Geometry check sheet. Reference: the model listing, model coordinates, mm. Face numbers are marked on the shaded views. A direction names the side the tool comes from. Give positions to 0.01 mm unless a question says otherwise; leave off trailing zeros. Write each loop counter-clockwise with the first axis right and the second up, starting at its lowest first coordinate (ties: lowest second). Pieces come first, ordered by that corner, then holes. Notation, with made-up numbers: (33, 75) - (83, 75) arc R36 ccw to (83, 109) - close; hole circle Ø7 at (60, 34.25). An arc over 180 degrees is marked (long way). Use a Markdown table: item, result.
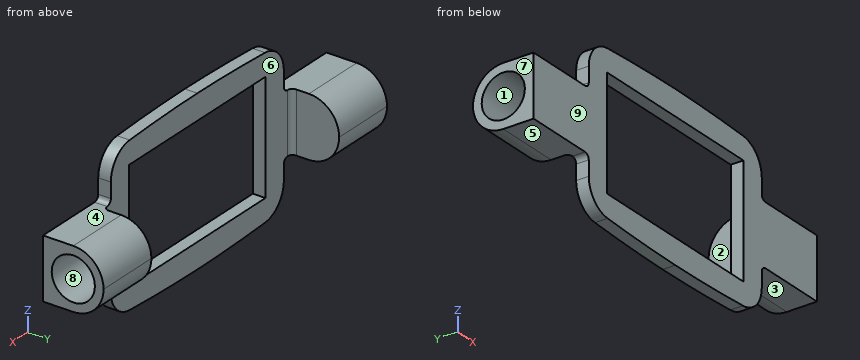
```python
from build123d import *

# Parameters (mm, degrees)
SKETCH2_W           = 93.98
SKETCH2_H           = 55.88
BOSS_EXTRUDE1_DEPTH = 6.35
SKETCH3_W           = 33.02
SKETCH3_H           = 30.48
BOSS_EXTRUDE2_DEPTH = 24.13
FILLET1_R           = 2.54
SKETCH4_R           = 10.8585
CUT_EXTRUDE1_DEPTH  = 25.4
CUT_EXTRUDE2_START  = -25.4
SKETCH5_R           = 10.8585
CUT_EXTRUDE2_DEPTH  = 25.4
FILLET2_R           = 2.54
FILLET3_R           = 15.24


with BuildPart() as part:
    # Sketch2 → Boss-Extrude1 (new body)
    with BuildSketch(Plane(origin=(0, 0, 0), x_dir=(1, 0, 0), z_dir=(0, 1, 0))):
        with BuildLine():
            ThreePointArc((-93.688069253, -11.244332686), (-70.349230661, -12.298232488), (-46.99, -12.696270789))
            ThreePointArc((-46.99, -12.696270789), (-23.630769339, -12.298232488), (-0.291930747, -11.244332686))
            ThreePointArc((-0.291930747, -11.244332686), (8.940138318, -6.930983214), (12.7, 2.54))
            Line((12.7, 2.54), (12.7, 12.7))
            Line((12.7, 12.7), (50.8, 12.7))
            Line((50.8, 12.7), (50.8, 43.18))
            Line((50.8, 43.18), (12.7, 43.18))
            Line((12.7, 43.18), (12.7, 53.34))
            ThreePointArc((12.7, 53.34), (8.940138318, 62.810983214), (-0.291930747, 67.124332686))
            ThreePointArc((-0.291930747, 67.124332686), (-23.630769339, 68.178232488), (-46.99, 68.576270789))
            ThreePointArc((-46.99, 68.576270789), (-70.349230661, 68.178232488), (-93.688069253, 67.124332686))
            ThreePointArc((-93.688069253, 67.124332686), (-102.920138318, 62.810983214), (-106.68, 53.34))
            Line((-106.68, 53.34), (-106.68, 43.18))
            Line((-106.68, 43.18), (-144.78, 43.18))
            Line((-144.78, 43.18), (-144.78, 12.7))
            Line((-144.78, 12.7), (-106.68, 12.7))
            Line((-106.68, 12.7), (-106.68, 2.54))
            ThreePointArc((-106.68, 2.54), (-102.920138318, -6.930983214), (-93.688069253, -11.244332686))
        make_face()
        with Locations((-46.99, 27.94)):
            Rectangle(SKETCH2_W, SKETCH2_H, mode=Mode.SUBTRACT)
    extrude(amount=BOSS_EXTRUDE1_DEPTH)

    # Sketch3 → Boss-Extrude2 (add)
    with BuildSketch(Plane(origin=(0, 6.35, 0), x_dir=(1, 0, 0), z_dir=(0, 1, 0))):
        with Locations((34.29, 27.94)):
            Rectangle(SKETCH3_W, SKETCH3_H)
        with Locations((-128.27, 27.94)):
            Rectangle(SKETCH3_W, SKETCH3_H)
    extrude(amount=BOSS_EXTRUDE2_DEPTH)

    # Fillet1
    fillet1_edges = [part.edges().sort_by_distance(p)[0] for p in [
        (17.78, 6.35, -27.94),
        (-111.76, 6.35, -27.94),
    ]]
    fillet(fillet1_edges, radius=FILLET1_R)

    # Sketch4 → Cut-Extrude1 (cut)
    with BuildSketch(Plane(origin=(50.8, 0, 0), x_dir=(0, 0, -1), z_dir=(1, 0, 0))):
        with Locations((27.94, 15.24)):
            Circle(SKETCH4_R)
    extrude(amount=-CUT_EXTRUDE1_DEPTH, mode=Mode.SUBTRACT)

    # Sketch5 → Cut-Extrude2 (cut)
    with BuildSketch(Plane.ZY.offset(144.78).offset(CUT_EXTRUDE2_START)):
        with Locations(Location((-27.94, 15.24, 0), (0, 0, 180))):
            Circle(SKETCH5_R)
    extrude(amount=CUT_EXTRUDE2_DEPTH, mode=Mode.SUBTRACT)

    # Fillet2
    fillet2_edges = [part.edges().sort_by_distance(p)[0] for p in [
        (12.7, 3.175, -43.18),
        (12.7, 3.175, -12.7),
        (-106.68, 3.175, -43.18),
        (-106.68, 3.175, -12.7),
    ]]
    fillet(fillet2_edges, radius=FILLET2_R)

    # Fillet3
    fillet3_edges = [part.edges().sort_by_distance(p)[0] for p in [
        (34.29, 30.48, -43.18),
        (34.29, 30.48, -12.7),
        (-128.27, 30.48, -43.18),
        (-128.27, 30.48, -12.7),
    ]]
    fillet(fillet3_edges, radius=FILLET3_R - 0.0001)  # a hair under: the kernel refuses the full size


solid = part.part
```
1) Material ranges on L1, parallel to X at y = 9.5, z = -25; L2, parallel to Y at x = 34.25, z = -27.94; L3, parallel to Z at x = 39, y = 15, recorded low to high. Write a range as from..to.
Working result:
| item | result |
|---|---|
| L1 | x = -119.38..-111.76, 17.78..25.4 |
| L2 | y = 0..4.38, 26.1..30.48 |
| L3 | z = -43.18..-38.8, -17.08..-12.7 |
2) Section check D-D on x = -61. Record the boundary of the cut face in (y, z).
Working result:
| item | result |
|---|---|
| outline | (0, -68.42) - (6.35, -68.42) - (6.35, -55.88) - (0, -55.88) - close; (0, 0) - (6.35, 0) - (6.35, 12.54) - (0, 12.54) - close |
3) Mould release check, pull along Y, two halves, no side actions. Record for the marked faces 6, 7, 8 and 9: pulls with the +Y half, pulls with the -Y half, needs draft (parallel to the pull), parting line crosses it, or undercut.
Working result:
| item | result |
|---|---|
| face 6 | pulls with the +Y half |
| face 7 | needs draft |
| face 8 | undercut |
| face 9 | pulls with the -Y half |
4) Set-up check for the marked faces 1, 2, 3, 4 and 5: record each of +Z, -Z, +X, -X, +Y, -Y from which the full face is reachable in a straight line by a thin tool's end or side.
Working result:
| item | result |
|---|---|
| face 1 | -X |
| face 2 | +Z, -Z, +Y |
| face 3 | -Z, +X, +Y, -Y |
| face 4 | +Z, +X, +Y, -Y |
| face 5 | -Z, -X, +Y, -Y |
5) Depth check by flat-ended pin: P1, Ø24.5, axis at x = -18.5, z = -46.5, coming from the +Y side; P2, Ø4.5, axis at x = 29, y = 8, coming from the -Z side; P3, Ø7, axis at y = 2.5, z = -5, coming from the +X side. Enter the tip coordinate at first touch or a pass-through.
Working result:
| item | result |
|---|---|
| P1 | stops at y = 6.35 |
| P2 | stops at z = -43.18 |
| P3 | stops at x = 12.7 |
6) Section check C-C on y = 19. Record the boundary of the cut face in (x, z), then the cut area to 3 significant figures.
Working result:
| item | result |
|---|---|
| outline | (-144.78, -42.71) - (-111.76, -42.71) - (-111.76, -13.17) - (-144.78, -13.17) - (-144.78, -17.75) - (-119.38, -17.75) - (-119.38, -38.13) - (-144.78, -38.13) - close; (17.78, -42.71) - (50.8, -42.71) - (50.8, -38.13) - (25.4, -38.13) - (25.4, -17.75) - (50.8, -17.75) - (50.8, -13.17) - (17.78, -13.17) - close |
| area | 916 mm² |
7) Section check A-A on z = -4.5. Record the boundary of the cut face in (x, y), then the cut area to 3 significant figures.
Working result:
| item | result |
|---|---|
| outline | (-106.68, 0) - (-93.98, 0) - (-93.98, 6.35) - (-106.68, 6.35) - close; (0, 0) - (12.7, 0) - (12.7, 6.35) - (0, 6.35) - close |
| area | 161 mm² |
